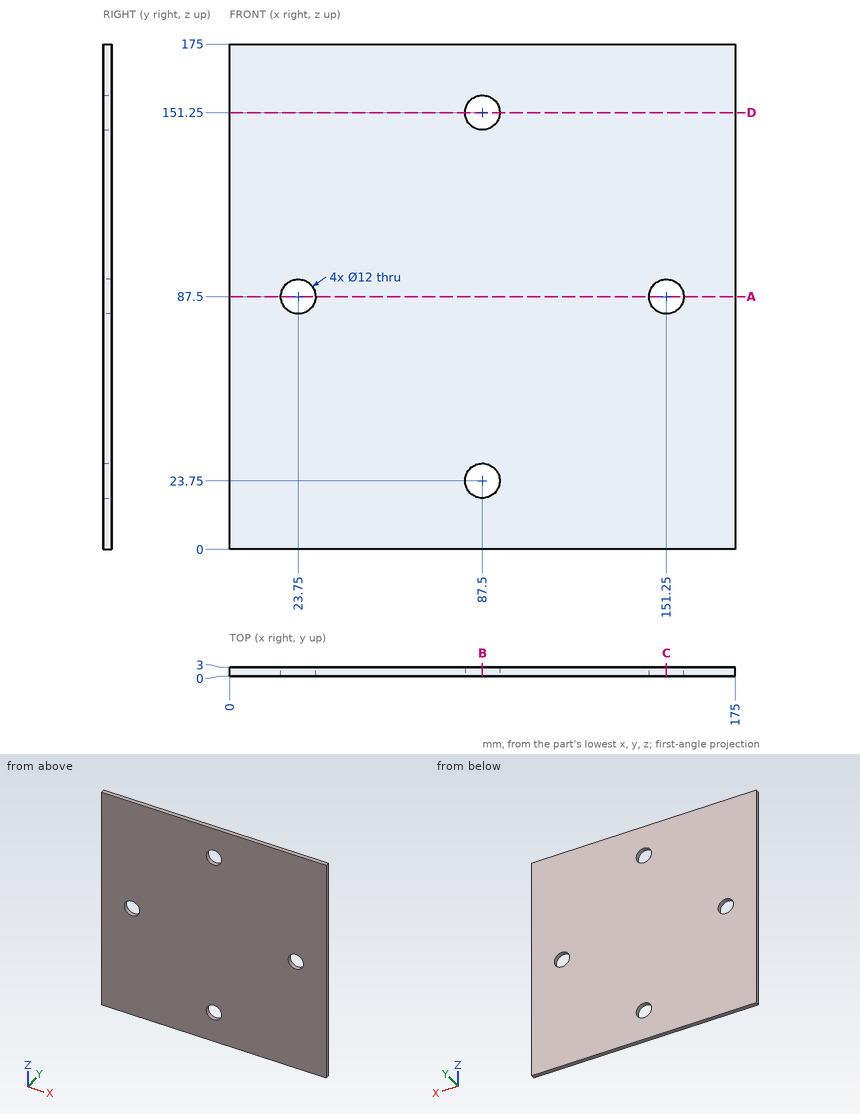
Job drawing, mm, ordinate dimensions from the low corner. One solid piece. Round coordinates to 2 decimals unless told otherwise and drop trailing zeros. Loops run counter-clockwise (first coordinate to the right, second up) from the corner with the lowest first, then second, coordinate; pieces in that order, holes last. Notation, with made-up numbers: (52, 53.25) -> (104, 53.25) arc R25 cw to (104, 67.25) -> close; hole circle Ø8 at (62, -0.75). An arc over 180 degrees is marked (long way). Use CSV: the item, a comma, the result in double quotes. Start each with the question number.
Q1. Saw through at D-D on z = 151.25. Give the cut face in (x, y).
Q2. Saw through at B-B on x = 87.5. Give the cut face in (y, z).
Q3. Drill centre lines: L1, parallel to Z at x = 87.5, y = 0.95; L2, parallel to X at y = 2.25, z = 91. Where is each one in solid material? Low to high.
Q4. Saw through at C-C on x = 151.25. Give the cut face in (y, z), and give its area (3 significant figures).
Q5. Saw through at A-A on z = 87.5. Give the cut face in (x, y).
Solutions:
1,outline,"(0, 0) -> (81.5, 0) -> (81.5, 3) -> (0, 3) -> close; (93.5, 0) -> (175, 0) -> (175, 3) -> (93.5, 3) -> close"
2,outline,"(0, 0) -> (3, 0) -> (3, 17.75) -> (0, 17.75) -> close; (0, 29.75) -> (3, 29.75) -> (3, 145.25) -> (0, 145.25) -> close; (0, 157.25) -> (3, 157.25) -> (3, 175) -> (0, 175) -> close"
3,L1,"z = 0 to 17.75, 29.75 to 145.25, 157.25 to 175"
3,L2,"x = 0 to 18.88, 28.62 to 146.38, 156.12 to 175"
4,outline,"(0, 0) -> (3, 0) -> (3, 81.5) -> (0, 81.5) -> close; (0, 93.5) -> (3, 93.5) -> (3, 175) -> (0, 175) -> close"
4,area,"489 mm^2"
5,outline,"(0, 0) -> (17.75, 0) -> (17.75, 3) -> (0, 3) -> close; (29.75, 0) -> (145.25, 0) -> (145.25, 3) -> (29.75, 3) -> close; (157.25, 0) -> (175, 0) -> (175, 3) -> (157.25, 3) -> close"
